The listing builds one solid part. Answer for the finished solid, in the listing's coordinates (mm). Face numbers are marked on the shaded views. Round coordinates to 2 decimals unless told otherwise and drop trailing zeros. Order: outer loops, then holes, each group sorted by start corner. A loop starts at its lowest first (then second) coordinate and runs counter-clockwise, first axis right, second up. Notation, with made-up numbers: (41.25, 62) - (65.25, 62) arc R20 cw to (65.25, 74) - close; hole circle Ø9 at (-12.5, 20.5). An arc over 180 degrees is marked (long way). One line per item, written item: value. Start each with the question number.
1. Straight lines are drawn through the part: line 1 (X direction, y = 10.5, z = 0); line 2 (X direction, y = 9.5, z = -10); line 3 (Y direction, x = 40, z = 25). For each, find the intervals that lie inside material, in ascending order.
2. Section D-D, the plane y = 16.5 is taken. Give the vertices of the cut face in (x, z), then the cut area to 3 significant figures.
3. Flat-ended cylindrical pins translate along their axes: P1, Ø8, axis at y = 3.5, z = 34.5, coming from the -X side; P2, Ø5, axis at y = 2, z = -18, coming from the -X side; P3, Ø1.8, axis at x = 0, z = -48, coming from the +Y side; P4, Ø1.5, axis at x = -29, y = 6.5, coming from the +Z side. Find the tip coordinate at first contact, or state that the pin passes through.
4. Section B-B, the plane x = 19 is taken. Give the vertices of the cut face in (y, z), then the cut area to 3 significant figures.
5. Section A-A, the plane z = 0 is taken. Give the vertices of the cut face in (x, y).
6. For a pull along Z with two mould halves and no side action, classify the marked faces 1, 2 and 3 as released by +Z, released by -Z, zero draft, split by the parting line, or undercut.
7. Section C-C, the plane z = -33.5 is taken. Give the vertices of the cut face in (x, y).
from build123d import *

# Parameters (mm, degrees)
SKETCH1_R           = 45
SKETCH1_R_2         = 42
BOSS_EXTRUDE1_DEPTH = 20
SKETCH2_R           = 51
SKETCH2_R_2         = 1.5
SKETCH2_R_3         = 45
BOSS_EXTRUDE2_DEPTH = 5
BOSS_EXTRUDE3_START = -20
SKETCH3_R           = 42
SKETCH3_R_2         = 41.5
BOSS_EXTRUDE3_DEPTH = 20
SKETCH4_R           = 41.7
SKETCH4_R_2         = 41.5
CUT_EXTRUDE1_DEPTH  = 75.846509605


with BuildPart() as part:
    # Sketch1 → Boss-Extrude1 (new body)
    with BuildSketch(Plane(origin=(0, 0, 0), x_dir=(1, 0, 0), z_dir=(0, 1, 0))):
        with Locations(Location((0, 0, 0), (0, 0, 270))):
            Circle(SKETCH1_R)
        with Locations(Location((0, 0, 0), (0, 0, 270))):
            Circle(SKETCH1_R_2, mode=Mode.SUBTRACT)
    extrude(amount=BOSS_EXTRUDE1_DEPTH)

    # Sketch2 → Boss-Extrude2 (add)
    with BuildSketch(Plane.XZ):
        with Locations(Location((0, 0, 0), (0, 0, 270))):
            Circle(SKETCH2_R)
        with Locations(Location((0, -48, 0), (0, 0, 270))):
            Circle(SKETCH2_R_2, mode=Mode.SUBTRACT)
        with Locations(Location((-48, 0, 0), (0, 0, 270))):
            Circle(SKETCH2_R_2, mode=Mode.SUBTRACT)
        with Locations(Location((0, 0, 0), (0, 0, 270))):
            Circle(SKETCH2_R_3, mode=Mode.SUBTRACT)
        with BuildLine():
            ThreePointArc((49.5, 0), (48, -1.5), (46.5, 0))
            ThreePointArc((46.5, 0), (48, 1.5), (49.5, 0))
        make_face(mode=Mode.SUBTRACT)
        with Locations(Location((0, 48, 0), (0, 0, 270))):
            Circle(SKETCH2_R_2, mode=Mode.SUBTRACT)
    extrude(amount=-BOSS_EXTRUDE2_DEPTH)

    # Sketch3 → Boss-Extrude3 (add)
    with BuildSketch(Plane(origin=(0, 20, 0), x_dir=(1, 0, 0), z_dir=(0, 1, 0)).offset(BOSS_EXTRUDE3_START)):
        Circle(SKETCH3_R)
        with Locations(Location((0, 0, 0), (0, 0, 270))):
            Circle(SKETCH3_R_2, mode=Mode.SUBTRACT)
    extrude(amount=BOSS_EXTRUDE3_DEPTH)

    # Sketch4 → Cut-Extrude1 (cut, through all)
    with BuildSketch(Plane(origin=(0, 20, 0), x_dir=(1, 0, 0), z_dir=(0, 1, 0))):
        with Locations(Location((0, 0, 0), (0, 0, 270))):
            Circle(SKETCH4_R)
        Circle(SKETCH4_R_2, mode=Mode.SUBTRACT)
    extrude(amount=-CUT_EXTRUDE1_DEPTH, mode=Mode.SUBTRACT)


solid = part.part
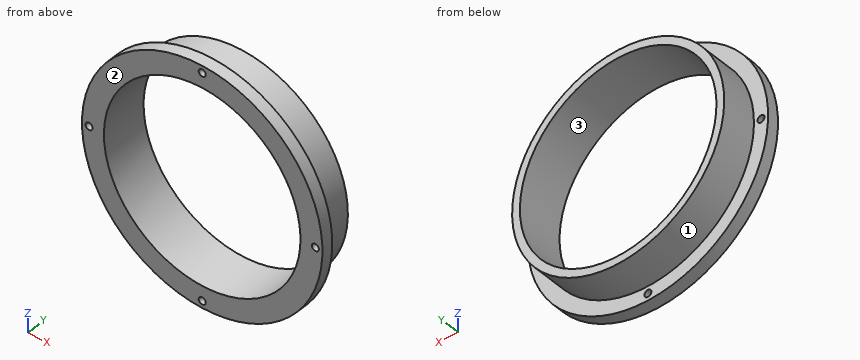
Answer list:
1. line 1: x = -45 to -41.7, 41.7 to 45
1. line 2: x = -43.87 to -40.48, 40.48 to 43.87
1. line 3: y = 0 to 5
2. outline: circle Ø90 at (0, 0); hole circle Ø83.4 at (0, 0)
2. area: 899 mm²
3. P1: stops at x = -40.87
3. P2: stops at x = -48.59
3. P3: passes through
3. P4: stops at z = 35.03
4. outline: (0, -47.33) - (5, -47.33) - (5, -40.79) - (20, -40.79) - (20, -37.12) - (0, -37.12) - close; (0, 37.12) - (20, 37.12) - (20, 40.79) - (5, 40.79) - (5, 47.33) - (0, 47.33) - close
4. area: 212 mm²
5. outline: (-51, 0) - (-49.5, 0) - (-49.5, 5) - (-51, 5) - close; (-46.5, 0) - (-41.7, 0) - (-41.7, 20) - (-45, 20) - (-45, 5) - (-46.5, 5) - close; (41.7, 0) - (46.5, 0) - (46.5, 5) - (45, 5) - (45, 20) - (41.7, 20) - close; (49.5, 0) - (51, 0) - (51, 5) - (49.5, 5) - close
6. face 1: split by the parting line
6. face 2: zero draft
6. face 3: undercut
7. outline: (-38.45, 0) - (-24.83, 0) - (-24.83, 20) - (-30.05, 20) - (-30.05, 5) - (-38.45, 5) - close; (24.83, 0) - (38.45, 0) - (38.45, 5) - (30.05, 5) - (30.05, 20) - (24.83, 20) - close
